Work out the finished part from the listing and answer in its coordinate system (mm). Round coordinates to 2 decimals unless told otherwise and drop trailing zeros. Write each loop counter-clockwise with the first axis right and the second up, starting at its lowest first coordinate (ties: lowest second). Pieces come first, ordered by that corner, then holes.
1. Straight lines are drawn through the part: probe 1 along X at (y, z) = (4.5, -50); probe 2 along X at (y, z) = (2.25, -112); probe 3 along Z at (x, y) = (117, 6) (3 decimals). For each, find the intervals that lie inside material, in ascending order.
2. A flat-ended cylindrical pin translates along its axis: pin 1 Ø6 at (x, z) = (76.2, -12.7) entering from -Y. Find the tip coordinate at first contact, or state that the pin passes through.
3. Find section B-B (y = 4). Count the separate pieces of the cut face and the enclosed holes in it, and give its area (3 significant figures).
4. Find section A-A (z = -100). Write down the section's boundary in (x, y), and give its area (3 significant figures).
```python
from build123d import *

# Parameters (mm, degrees)
SKETCH2_W           = 609.6
SKETCH2_H           = 152.4
BOSS_EXTRUDE1_DEPTH = 6.35
CUT_EXTRUDE1_REACH  = 630.393
SKETCH3_W           = 50.8
SKETCH3_H           = 82.55
SKETCH4_R           = 3.3782
CUT_EXTRUDE2_DEPTH  = 629.393381967
SKETCH5_R           = 3.3782
CUT_EXTRUDE3_DEPTH  = 629.393381967
SKETCH6_R           = 3.3782
CUT_EXTRUDE4_DEPTH  = 629.393381967


with BuildPart() as part:
    # Sketch2 → Boss-Extrude1 (new body)
    with BuildSketch(Plane(origin=(0, 0, 0), x_dir=(1, 0, 0), z_dir=(0, 1, 0))):
        with Locations((304.8, 76.2)):
            Rectangle(SKETCH2_W, SKETCH2_H)
    extrude(amount=BOSS_EXTRUDE1_DEPTH)

    # Sketch3 → Cut-Extrude1 (cut, up to next)
    with BuildSketch(Plane(origin=(0, 6.35, 0), x_dir=(1, 0, 0), z_dir=(0, 1, 0)), mode=Mode.PRIVATE) as cut_extrude1_sk1:
        with Locations((119.1006, 76.2)):
            Rectangle(SKETCH3_W, SKETCH3_H)
    cut_extrude1_tool1 = extrude(cut_extrude1_sk1.sketch, amount=-CUT_EXTRUDE1_REACH, mode=Mode.PRIVATE) & part.part
    add(cut_extrude1_tool1.solids().sort_by_distance((119.1006, 6.35, -76.2))[0], mode=Mode.SUBTRACT)

    # Sketch4 → Cut-Extrude2 (cut, through all)
    with BuildSketch(Plane(origin=(0, 6.35, 0), x_dir=(1, 0, 0), z_dir=(0, 1, 0))):
        with Locations(Location((571.5, 12.7, 0), (0, 0, 270))):
            Circle(SKETCH4_R)
        with Locations(Location((571.5, 139.7, 0), (0, 0, 270))):
            Circle(SKETCH4_R)
        with Locations(Location((76.2, 12.7, 0), (0, 0, 270))):
            Circle(SKETCH4_R)
        with Locations(Location((76.2, 139.7, 0), (0, 0, 270))):
            Circle(SKETCH4_R)
    extrude(amount=-CUT_EXTRUDE2_DEPTH, mode=Mode.SUBTRACT)

    # Sketch5 → Cut-Extrude3 (cut, through all)
    with BuildSketch(Plane(origin=(0, 6.35, 0), x_dir=(1, 0, 0), z_dir=(0, 1, 0))):
        with Locations(Location((595.3125, 113.587796728, 0), (0, 0, 270))):
            Circle(SKETCH5_R)
        with Locations(Location((595.3125, 38.812203272, 0), (0, 0, 270))):
            Circle(SKETCH5_R)
        with Locations(Location((184.15, 38.812203272, 0), (0, 0, 270))):
            Circle(SKETCH5_R)
        with Locations(Location((184.15, 113.587796728, 0), (0, 0, 270))):
            Circle(SKETCH5_R)
    extrude(amount=-CUT_EXTRUDE3_DEPTH, mode=Mode.SUBTRACT)

    # Sketch6 → Cut-Extrude4 (cut, through all)
    with BuildSketch(Plane(origin=(0, 6.35, 0), x_dir=(1, 0, 0), z_dir=(0, 1, 0))):
        with Locations(Location((12.7, 36.14928, 0), (0, 0, 270))):
            Circle(SKETCH6_R)
        with Locations(Location((12.7, 10.74928, 0), (0, 0, 270))):
            Circle(SKETCH6_R)
        with Locations(Location((44.45, 10.74928, 0), (0, 0, 270))):
            Circle(SKETCH6_R)
        with Locations(Location((44.45, 36.14928, 0), (0, 0, 270))):
            Circle(SKETCH6_R)
        with Locations(Location((12.7, 141.65072, 0), (0, 0, 270))):
            Circle(SKETCH6_R)
        with Locations(Location((12.7, 116.25072, 0), (0, 0, 270))):
            Circle(SKETCH6_R)
        with Locations(Location((44.45, 116.25072, 0), (0, 0, 270))):
            Circle(SKETCH6_R)
        with Locations(Location((44.45, 141.65072, 0), (0, 0, 270))):
            Circle(SKETCH6_R)
    extrude(amount=-CUT_EXTRUDE4_DEPTH, mode=Mode.SUBTRACT)


solid = part.part
```
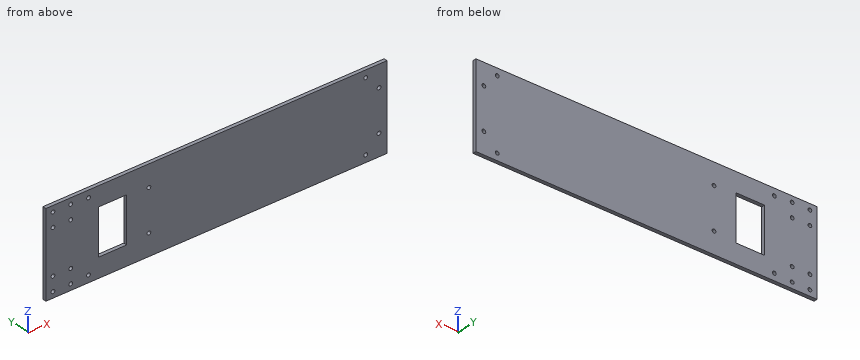
Worked answers:
1. probe 1: x = 0 to 93.7, 144.5 to 609.6
1. probe 2: x = 0 to 93.7, 144.5 to 181.17, 187.13 to 592.33, 598.29 to 609.6
1. probe 3: z = -152.4 to -117.475, -34.925 to 0
2. pin 1: passes through
3. separate pieces: 1
3. enclosed holes: 17
3. area: 88,100 mm2
4. outline: (0, 0) - (93.7, 0) - (93.7, 6.35) - (0, 6.35) - close; (144.5, 0) - (609.6, 0) - (609.6, 6.35) - (144.5, 6.35) - close
4. area: 3,550 mm2
